Read the model definition and answer for the solid it produces. Units are mm, in the model's axes. Face numbers are marked on the shaded views. Give positions to 0.01 mm unless a question says otherwise; leave off trailing zeros. Order: outer loops, then holes, each group sorted by start corner. A loop starts at its lowest first (then second) coordinate and runs counter-clockwise, first axis right, second up. Notation, with made-up numbers: (-20.5, 43.25) - (-11.5, 43.25) arc R19 ccw to (-11.5, 70.25) - close; hole circle Ø8 at (-14, 24). An arc over 180 degrees is marked (long way). Return JSON: item names as keys, results as strings.
```python
from build123d import *

# Parameters (mm, degrees)
SKETCH1_R            = 2.4
BEAM_DEPTH           = 3.925
SKETCH3_R            = 3.1
HOLE_SURROUND_DEPTH  = 1.25
CAVITY_CUT_DEPTH     = 3
FILLET2_R            = 0.5
FILLET2_OF_MIRROR2_R = 0.5


with BuildPart() as part:
    # Sketch1 → Beam (new, symmetric)
    with BuildSketch(Plane.XY):
        with BuildLine():
            Line((0, 3.7), (32, 3.7))
            ThreePointArc((32, 3.7), (35.7, 0), (32, -3.7))
            Line((32, -3.7), (0, -3.7))
            ThreePointArc((0, -3.7), (-3.7, 0), (0, 3.7))
        make_face()
        Circle(SKETCH1_R, mode=Mode.SUBTRACT)
        with Locations((8, 0)):
            Circle(SKETCH1_R, mode=Mode.SUBTRACT)
        with Locations((16, 0)):
            Circle(SKETCH1_R, mode=Mode.SUBTRACT)
        with Locations((24, 0)):
            Circle(SKETCH1_R, mode=Mode.SUBTRACT)
        with Locations((32, 0)):
            Circle(SKETCH1_R, mode=Mode.SUBTRACT)
    extrude(amount=BEAM_DEPTH, both=True)

    # Sketch3 → Hole Surround (cut)
    with BuildSketch(Plane.XY.offset(3.925)):
        with Locations((32, 0)):
            Circle(SKETCH3_R)
        with Locations((24, 0)):
            Circle(SKETCH3_R)
        with Locations((16, 0)):
            Circle(SKETCH3_R)
        with Locations((8, 0)):
            Circle(SKETCH3_R)
        Circle(SKETCH3_R)
    hole_surround = extrude(amount=-HOLE_SURROUND_DEPTH, mode=Mode.SUBTRACT)

    # Sketch4 → Cavity Cut (cut)
    with BuildSketch(Plane.XY.offset(3.925)):
        with BuildLine():
            ThreePointArc((3.65, 0), (3.338212028, -1.476089583), (2.456114818, -2.7))
            Line((2.456114818, -2.7), (5.543885182, -2.7))
            ThreePointArc((5.543885182, -2.7), (4.35, 0), (5.543885182, 2.7))
            Line((5.543885182, 2.7), (2.456114818, 2.7))
            ThreePointArc((2.456114818, 2.7), (3.338212028, 1.476089583), (3.65, 0))
        make_face()
        with BuildLine():
            ThreePointArc((11.65, 0), (11.338212028, -1.476089583), (10.456114818, -2.7))
            Line((10.456114818, -2.7), (13.543885182, -2.7))
            ThreePointArc((13.543885182, -2.7), (12.35, 0), (13.543885182, 2.7))
            Line((13.543885182, 2.7), (10.456114818, 2.7))
            ThreePointArc((10.456114818, 2.7), (11.338212028, 1.476089583), (11.65, 0))
        make_face()
        with BuildLine():
            ThreePointArc((19.65, 0), (19.338212028, -1.476089583), (18.456114818, -2.7))
            Line((18.456114818, -2.7), (21.543885182, -2.7))
            ThreePointArc((21.543885182, -2.7), (20.35, 0), (21.543885182, 2.7))
            Line((21.543885182, 2.7), (18.456114818, 2.7))
            ThreePointArc((18.456114818, 2.7), (19.338212028, 1.476089583), (19.65, 0))
        make_face()
        with BuildLine():
            ThreePointArc((27.65, 0), (27.338212028, -1.476089583), (26.456114818, -2.7))
            Line((26.456114818, -2.7), (29.543885182, -2.7))
            ThreePointArc((29.543885182, -2.7), (28.35, 0), (29.543885182, 2.7))
            Line((29.543885182, 2.7), (26.456114818, 2.7))
            ThreePointArc((26.456114818, 2.7), (27.338212028, 1.476089583), (27.65, 0))
        make_face()
    cavity_cut = extrude(amount=-CAVITY_CUT_DEPTH, mode=Mode.SUBTRACT)

    # Fillet2
    fillet2_edges = [part.edges().sort_by_distance(p)[0] for p in [
        (2.456114818, -2.7, 2.425),
        (2.456114818, 2.7, 2.425),
        (5.543885182, 2.7, 2.425),
        (5.543885182, -2.7, 2.425),
        (10.456114818, -2.7, 2.425),
        (10.456114818, 2.7, 2.425),
        (13.543885182, 2.7, 2.425),
        (13.543885182, -2.7, 2.425),
        (18.456114818, -2.7, 2.425),
        (18.456114818, 2.7, 2.425),
        (21.543885182, 2.7, 2.425),
        (21.543885182, -2.7, 2.425),
        (26.456114818, -2.7, 2.425),
        (26.456114818, 2.7, 2.425),
        (29.543885182, 2.7, 2.425),
        (29.543885182, -2.7, 2.425),
    ]]
    fillet(fillet2_edges, radius=FILLET2_R)

    # Mirror2: Hole Surround, Cavity Cut across plane
    add(hole_surround.mirror(Plane.XY), mode=Mode.SUBTRACT)
    add(cavity_cut.mirror(Plane.XY), mode=Mode.SUBTRACT)

    # Fillet2 of Mirror2
    fillet2_of_mirror2_edges = [part.edges().sort_by_distance(p)[0] for p in [
        (2.456114818, -2.7, -2.425),
        (2.456114818, 2.7, -2.425),
        (5.543885182, 2.7, -2.425),
        (5.543885182, -2.7, -2.425),
        (10.456114818, -2.7, -2.425),
        (10.456114818, 2.7, -2.425),
        (13.543885182, 2.7, -2.425),
        (13.543885182, -2.7, -2.425),
        (18.456114818, -2.7, -2.425),
        (18.456114818, 2.7, -2.425),
        (21.543885182, 2.7, -2.425),
        (21.543885182, -2.7, -2.425),
        (26.456114818, -2.7, -2.425),
        (26.456114818, 2.7, -2.425),
        (29.543885182, 2.7, -2.425),
        (29.543885182, -2.7, -2.425),
    ]]
    fillet(fillet2_of_mirror2_edges, radius=FILLET2_OF_MIRROR2_R)


solid = part.part
```
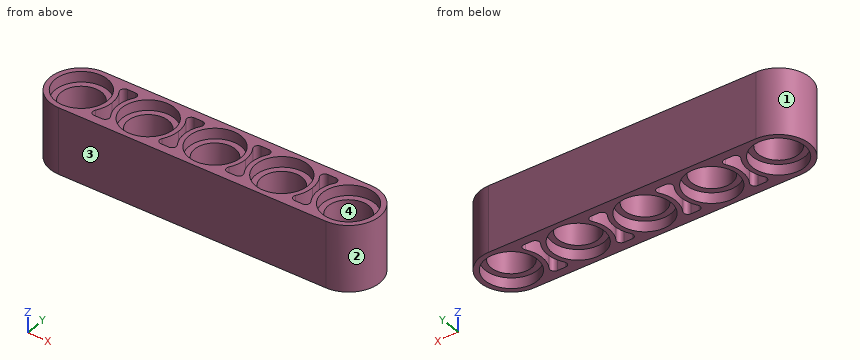
Q1. A cutting plane is placed at D-D (y = 1.25). Give the number of separate pieces and of enclosed holes in the cut face, and give its area (4 significant figures).
Values:
{"separate pieces": "6", "enclosed holes": "0", "area": "97.95 mm²"}
Q2. A cutting plane is placed at A-A (z = 0.5). Write down the section's boundary in (x, y), and give its area (3 significant figures).
Values:
{"outline": "(0, -3.7) - (32, -3.7) arc R3.7 ccw to (32, 3.7) - (0, 3.7) arc R3.7 ccw to start; hole circle Ø4.8 at (0, 0); hole circle Ø4.8 at (8, 0); hole circle Ø4.8 at (16, 0); hole circle Ø4.8 at (24, 0); hole circle Ø4.8 at (32, 0)", "area": "189 mm²"}
Q3. Determine the mould class of the marked faces 1, 2, 3 and 4 for opening direction X: released by +X, released by -X, zero draft, split by the parting line, or undercut.
Values:
{"face 1": "released by -X", "face 2": "released by +X", "face 3": "zero draft", "face 4": "undercut"}
Q4. Given pin 1 (1 mm diameter, centred on y = -1.5, z = 1, fed in from -X), flat-ended and moving along its own axis, determine where the tip first touches the part or whether it passes through.
Values:
{"pin 1": "stops at x = -3.56"}
Q5. Consider L1, parallel to X at y = 0, z = 0.75; L2, parallel to Y at x = 16, z = 2.5; L3, parallel to Y at x = 8, z = -2.95. Determine where each line is inside the solid, lowest interval first.
Values:
{"L1": "x = -3.7 to -2.4, 2.4 to 5.6, 10.4 to 13.6, 18.4 to 21.6, 26.4 to 29.6, 34.4 to 35.7", "L2": "y = -3.7 to -2.4, 2.4 to 3.7", "L3": "y = -3.7 to -3.1, 3.1 to 3.7"}
Q6. A cutting plane is placed at B-B (x = 16). Write down the section's boundary in (y, z) (3 decimals).
Values:
{"outline": "(-3.7, -3.925) - (-3.1, -3.925) - (-3.1, -2.675) - (-2.4, -2.675) - (-2.4, 2.675) - (-3.1, 2.675) - (-3.1, 3.925) - (-3.7, 3.925) - close; (2.4, -2.675) - (3.1, -2.675) - (3.1, -3.925) - (3.7, -3.925) - (3.7, 3.925) - (3.1, 3.925) - (3.1, 2.675) - (2.4, 2.675) - close"}
Q7. A cutting plane is placed at C-C (x = 12). Write down the section's boundary in (y, z) (3 decimals), and give its area (3 significant figures).
Values:
{"outline": "(-3.7, -3.925) - (-2.7, -3.925) - (-2.7, -0.925) - (2.7, -0.925) - (2.7, -3.925) - (3.7, -3.925) - (3.7, 3.925) - (2.7, 3.925) - (2.7, 0.925) - (-2.7, 0.925) - (-2.7, 3.925) - (-3.7, 3.925) - close", "area": "25.7 mm²"}
